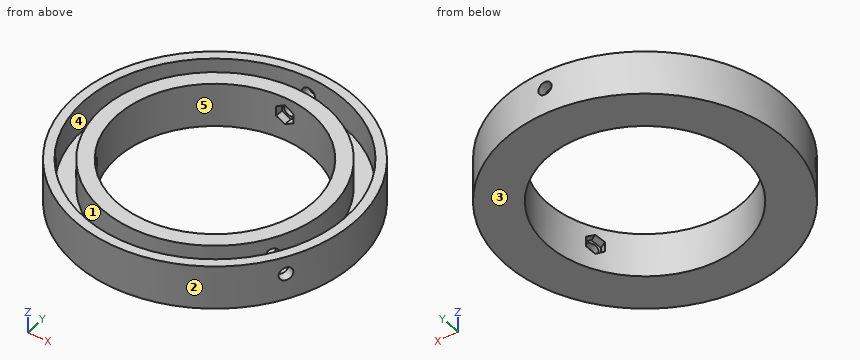
from build123d import *

# Parameters (mm, degrees)
F0_R             = 38.5
F0_R_2           = 33.35
F1_DEPTH         = 15
F2_R             = 44.5
F2_R_2           = 38.5
F3_DEPTH         = 5
F4_R             = 47.7
F4_R_2           = 44.5
F5_DEPTH         = 15
F6_R             = 2.25
F7_DEPTH         = 47.701
F7_COPIES_COUNT  = 3
F10_DEPTH        = 4
F10_COPIES_COUNT = 3


# Not quite as in the source:
# - a pattern or mirror of a feature is missing from the dataset's text; its kind, count and spacing are read off the source's solid


with BuildPart() as f1:
    # F0 (on Top) → F1 (new body)
    with BuildSketch(Plane.XY):
        Circle(F0_R)
        Circle(F0_R_2, mode=Mode.SUBTRACT)
    extrude(amount=F1_DEPTH)

    # F2 (on Top) → F3 (join)
    with BuildSketch(Plane.XY):
        Circle(F2_R)
        Circle(F2_R_2, mode=Mode.SUBTRACT)
    extrude(amount=F3_DEPTH)

    # F4 (on Top) → F5 (join)
    with BuildSketch(Plane.XY):
        Circle(F4_R)
        Circle(F4_R_2, mode=Mode.SUBTRACT)
    extrude(amount=F5_DEPTH)

    # F6 (on Front) → F7 (cut, through all)
    with BuildSketch(Plane.XZ):
        with Locations((0, 9)):
            Circle(F6_R)
    f7 = extrude(amount=-F7_DEPTH, mode=Mode.SUBTRACT)

    # F7_copies: F7 ×3 about axis
    f7_copies_axis = Axis((0, 0, 0), (0, 0, 1))
    for i in range(1, F7_COPIES_COUNT):
        add(f7.rotate(f7_copies_axis, i * 360 / F7_COPIES_COUNT), mode=Mode.SUBTRACT)

    # F9 (on offset) → F10 (cut)
    with BuildSketch(Plane.XZ.offset(-36)):
        Polygon((2.9175, 7.3155805896), (2.9175, 10.6844194104), (0, 12.3688388207), (-2.9175, 10.6844194104), (-2.9175, 7.3155805896), (0, 5.6311611793), align=None)
    f10 = extrude(amount=F10_DEPTH, mode=Mode.SUBTRACT)

    # F10_copies: F10 ×3 about axis
    f10_copies_axis = Axis((0, 0, 0), (0, 0, 1))
    for i in range(1, F10_COPIES_COUNT):
        add(f10.rotate(f10_copies_axis, i * 360 / F10_COPIES_COUNT), mode=Mode.SUBTRACT)


solid = f1.part
Input: part model. Units: mm. Frame: model coordinates. Face numbers are marked on the shaded views. A direction names the side the tool comes from. Round coordinates to 2 decimals unless told otherwise and drop trailing zeros. Order: outer loops, then holes, each group sorted by start corner. A loop starts at its lowest first (then second) coordinate and runs counter-clockwise, first axis right, second up. Notation, with made-up numbers: (37.25, -16) - (47.25, -16) arc R9 cw to (47.25, -9) - close; hole circle Ø1 at (11, 52). An arc over 180 degrees is marked (long way). Answer as a JSON object with one key per item and string values. Group by question number.
(1) Cut plane D-D (z = 9). Count the separate pieces of the cut face and the enclosed holes in it, then the cut area to 3 significant figures.
(2) Cut plane B-B (x = -18). Return loops of the section in (y, z), then the cut area to 3 significant figures.
(3) Draft query along X for the marked faces 1, 2 and 3. Return one class per face: released by +X, released by -X, zero draft, split by the parting line, or undercut.
(4) Cut plane C-C (z = 3.25). Return loops of the section in (x, y), then the cut area to 3 significant figures.
(5) Cut plane A-A (y = 0). Return loops of the section in (x, z), then the cut area to 4 significant figures.
(6) Pin query (flat end, axial travel): P1, Ø3, axis at x = -1, z = 6.5, coming from the -Y side; P2, Ø1.4, axis at y = 34.5, z = 9.5, coming from the -X side; P3, Ø0.8, axis at y = 35, z = 9, coming from the +X side. Return the tip coordinate at first contact, or that it passes through.
(7) Material intervals for probe 1 along X at (y, z) = (-1, 9) (3 decimals); probe 2 along X at (y, z) = (-7, 13); probe 3 along Y at (x, z) = (0, 7), sorted ascending. Write a range as from..to.
(8) Reachability of the marked faces 4 and 5 from +Z, -Z, +X, -X, +Y, -Y: full face, straight path, thin tool, end or side. Return the list, or none.
Here are the results:
{
 "1": {"separate pieces": "6", "enclosed holes": "0", "area": "1,970 mm^2"},
 "2": {"outline": "(-44.17, 0) - (-28.08, 0) - (-28.08, 15) - (-34.03, 15) - (-34.03, 5) - (-40.7, 5) - (-40.7, 15) - (-44.17, 15) - close; (28.08, 0) - (44.17, 0) - (44.17, 15) - (40.7, 15) - (40.7, 5) - (34.03, 5) - (34.03, 15) - (28.08, 15) - close", "area": "350 mm^2"},
 "3": {"face 1": "undercut", "face 2": "split by the parting line", "face 3": "zero draft"},
 "4": {"outline": "circle Ø95.4 at (0, 0); hole circle Ø66.7 at (0, 0)", "area": "3,650 mm^2"},
 "5": {"outline": "(-47.7, 0) - (-33.35, 0) - (-33.35, 15) - (-38.5, 15) - (-38.5, 5) - (-44.5, 5) - (-44.5, 15) - (-47.7, 15) - close; (33.35, 0) - (47.7, 0) - (47.7, 15) - (44.5, 15) - (44.5, 5) - (38.5, 5) - (38.5, 15) - (33.35, 15) - close", "area": "310.5 mm^2"},
 "6": {"P1": "stops at y = -47.7", "P2": "stops at x = -33.66", "P3": "stops at x = 32.83"},
 "7": {"probe 1": "x = -47.69..-44.489, -38.487..-33.335, 33.335..38.487, 44.489..47.69", "probe 2": "x = -47.18..-43.95, -37.86..-32.61, 32.61..37.86, 43.95..47.18", "probe 3": "y = -47.7..-44.5, -38.5..-33.35"},
 "8": {"face 4": "+Z", "face 5": "+Z, -Z"}
}
